Solid Edge part; units mm, degrees
sketch "Sketch1" plane through (0, 0, 0) normal (1, 0, 0) x (0, 1, 0)
  arc A0 (58.2893, 34.6118) -> (41.1893, 46.6809) centre (31.3554, 14.5992) ccw
  arc A1 (41.1893, 46.6809) -> (35.5, 54.3753) centre (43.5478, 54.3753) cw
  line L0 (35.5, 54.3753) -> (35.5, 56.9519)
  arc A2 (35.5, 56.9519) -> (39.1364, 60.9354) centre (39.5, 56.9519) cw
  arc A3 (39.1364, 60.9354) -> (48.5769, 58.6372) centre (40.5, 45.9975) cw
  arc A4 (48.5769, 58.6372) -> (49.5, 56.9519) centre (47.5, 56.9519) cw
  line L1 (49.5, 56.9519) -> (49.5, 51.9975)
  line L2 (49.5, 51.9975) -> (54.5, 51.9975)
  line L3 (54.5, 51.9975) -> (62.0448, 50.9602)
  arc A5 (62.0448, 50.9602) -> (65.5, 46.9975) centre (61.5, 46.9975) cw
  line L4 (65.5, 46.9975) -> (65.5, 36.9975)
  arc A6 (65.5, 36.9975) -> (58.2893, 34.6118) centre (61.5, 36.9975) cw
  circle A7 centre (61.5, 46.9975) radius 0.8
  circle A8 centre (61.5, 36.9975) radius 0.8
extrude "Protrusion1" add sketch "Sketch1" along normal mid plane 4
Verification items for the finished model (mm, model axes). A direction names the side the tool comes from. Give positions to 0.01 mm unless a question says otherwise; leave off trailing zeros. Write each loop counter-clockwise with the first axis right and the second up, starting at its lowest first coordinate (ties: lowest second). Pieces come first, ordered by that corner, then holes. Notation, with made-up numbers: M 27,35.5 L 61,35.5 A30 cw 61,60.5 Z; hole C 82,21.25 d1. An arc over 180 degrees is marked long. Put each result on its own line as item: value. Start each with the question number.
1. Draft check along Y on faces 3 (the face through (-0.028, 58.22, 51.486)), 4 (the face through (2, 50, 47)), 5 (the face through (-0.028, 62.263, 46.757)). Enter one of: +Y half, -Y half, draft (parallel to the pull), parting line (faces both ways), or undercut.
2. Go/stop test with flat-tipped pins: pin 1 Ø1 at (y, z) = (61.5, 47) entering from +X; pin 2 Ø1.2 at (x, y) = (-0.5, 51) entering from +Z; pin 3 Ø1 at (x, y) = (0, 58.5) entering from -Z (3 decimals). Record where each tip stops, or that it passes through.
3. Section check B-B (y = 61.5). Record the cut outline in (x, z), and give its area (3 significant figures).
4. Scan lines: line 1 along Z through (x, y) = (0.3, 61.5); line 2 along Z through (x, y) = (1.3, 62); line 3 along Y through (x, z) = (-1.35, 54.25). Record each from-to range of solid material in increasing order. Write a range as [from, to].
5. Set-up check for faces 1 (the face through (0, 65.5, 42)), 2 (the face through (0, 49.5, 55)): record each of +Z, -Z, +X, -X, +Y, -Y from which the full face is reachable in a straight line by a thin tool's end or side.
6. Section check C-C (z = 43.75). Record the cut outline in (x, y).
7. Section check D-D (y = 46.5). Record the cut outline in (x, z).
8. Section check A-A (x = 0.3). Record the cut outline in (y, z) (1 decimal), and give its area (3 significant figures).
Answer list:
1. face 3: +Y half
1. face 4: draft
1. face 5: undercut
2. pin 1: through
2. pin 2: z = 52
2. pin 3: z = 33.875
3. outline: M -2,33 L 2,33 L 2,36.2 L -2,36.2 Z; M -2,37.8 L 2,37.8 L 2,46.2 L -2,46.2 Z; M -2,47.8 L 2,47.8 L 2,51.04 L -2,51.04 Z
3. area: 59.4 mm2
4. line 1: [33, 36.2], [37.8, 46.2], [47.8, 51.04]
4. line 2: [33.03, 36.37], [37.62, 46.37], [47.62, 50.97]
4. line 3: [35.5, 49.5]
5. face 1: +Z, -Z, +X, -X, +Y
5. face 2: +Z, +X, -X, +Y
6. outline: M -2,47.97 L 2,47.97 L 2,65.5 L -2,65.5 Z
7. outline: M -2,44.54 L 2,44.54 L 2,59.75 L -2,59.75 Z
8. outline: M 35.5,54.4 A8 ccw 41.2,46.7 A33.6 cw 58.3,34.6 A4 ccw 65.5,37 L 65.5,47 A4 ccw 62,51 L 54.5,52 L 49.5,52 L 49.5,57 A2 ccw 48.6,58.6 A15 ccw 39.1,60.9 A4 ccw 35.5,57 Z; hole C 61.5,37 d1.6; hole C 61.5,47 d1.6
8. area: 420 mm2
